Can you work these out from the model? Positions are in its coordinate system, mm. A direction names the side the tool comes from. Round coordinates to 2 decimals unless told otherwise and drop trailing zeros. Write each loop counter-clockwise with the first axis right and the second up, starting at its lowest first coordinate (ties: lowest second). Pieces come first, ordered by that corner, then holes. Notation, with made-up numbers: M 27,76 L 41,76 A11 cw 41,94 Z; hole C 55,-29 d8. An arc over 180 degrees is marked long. Answer in a Markdown table with one row per item. Add a question column.
(1) If we mould it in two halves opening along Z, with no side actions, what happens to faces 1 (the face through (-39, 20.1, 10)), 2 (the face through (-15, 10, -2))? For each: released by +Z, released by -Z, zero draft, split by the parting line, or undercut.
(2) Suppose I cut it at D-D, the plane y = 22.25. Write out the boundary of the cut face in (x, z), then the cut area to 3 significant figures.
(3) Suppose I cut it at C-C, the plane x = -17.5. Write out the boundary of the cut face in (y, z).
(4) If I drill on probe 1 along Y at (x, z) = (-59, 19.25); probe 2 along Z at (x, y) = (-62, 2.5), over which ranges is the centre line in solid material (lowest first)?
(5) Suppose I cut it at B-B, the plane y = 10.05. Write out the boundary of the cut face in (x, z), then the cut area to 3 significant figures.
(6) Suppose I cut it at A-A, the plane z = 10.05. Write out the boundary of the cut face in (x, y).
(7) For faces 3 (the face through (-39.44, 4.48, 13.97)), 4 (the face through (-6, 22, 13.05)), 5 (the face through (-6, 7.05, -2)), 6 (the face through (-39, -4, 10)), 7 (the face through (-39, 24.1, 10)), which set-ups out of +Z, -Z, +X, -X, +Y, -Y let a thin tool reach every point of the face, with its end or its side?
Autodesk Inventor part; units mm, degrees
ref_plane "YZ Plane" through (0, 0, 0) normal (1, 0, 0) x (0, 1, 0)
ref_plane "XZ Plane" through (0, 0, 0) normal (0, 1, 0) x (-1, 0, 0)
ref_plane "XY Plane" through (0, 0, 0) normal (0, 0, 1) x (1, 0, 0)
sketch "Sketch1" plane through (0, 0, 0) normal (1, 0, 0) x (0, 1, 0)
  line L0 (0, 0) -> (20.1, 0)
  line L1 (20.1, 0) -> (20.1, 20.1)
  line L2 (20.1, 20.1) -> (0, 20.1)
  line L3 (0, 20.1) -> (0, 0)
  line L4 (-4, 24.1) -> (24.1, 24.1)
  line L5 (24.1, 24.1) -> (24.1, -4)
  line L6 (24.1, -4) -> (-4, -4)
  line L7 (-4, -4) -> (-4, 24.1)
  line L8 (12.55, 22.2) -> (7.55, 22.2)
  line L9 (7.55, 22.2) -> (7.55, 18)
  line L10 (7.55, 18) -> (12.55, 18)
  line L11 (12.55, 18) -> (12.55, 22.2)
  line L12 (12.55, 22.2) -> (7.55, 18) construction
  line L13 (7.55, 22.2) -> (12.55, 18) construction
  line L14 (12.55, 18) -> (15.35, 18)
  line L15 (15.35, 18) -> (15.35, 17)
  line L16 (15.35, 17) -> (12.55, 14.2)
  line L17 (12.55, 14.2) -> (7.55, 14.2)
  line L18 (7.55, 18) -> (4.75, 18)
  line L19 (4.75, 18) -> (4.75, 17)
  line L20 (4.75, 17) -> (7.55, 14.2)
  line L21 (2.1, 15.35) -> (3.1, 15.35)
  line L22 (3.1, 4.75) -> (5.9, 7.55)
  line L23 (2.1, 4.75) -> (3.1, 4.75)
  line L24 (-2.1, 12.55) -> (-2.1, 7.55)
  line L25 (2.1, 12.55) -> (-2.1, 12.55)
  line L26 (-2.1, 12.55) -> (2.1, 7.55) construction
  line L27 (-2.1, 7.55) -> (2.1, 12.55) construction
  line L28 (2.1, 7.55) -> (2.1, 4.75)
  line L29 (-2.1, 7.55) -> (2.1, 7.55)
  line L30 (2.1, 7.55) -> (2.1, 12.55)
  line L31 (5.9, 12.55) -> (5.9, 7.55)
  line L32 (2.1, 12.55) -> (2.1, 15.35)
  line L33 (3.1, 15.35) -> (5.9, 12.55)
  point P0 (10.05, 20.1)
  point P1 (0, 10.05)
  point P2 (10.05, 20.1)
  point P3 (0, 10.05)
  point P4 (0, 7.55)
  point P5 (0, 12.55)
  point P6 (7.55, 20.1)
  point P7 (12.55, 20.1)
  dimension "d0" = 20.1
  dimension "d1" = 20.1
  dimension "d2" = 4
  dimension "d3" = 5
  dimension "d4" = 4.2
  dimension "d5" = 2.8
  dimension "d6" = 1
  dimension "d7" = 3.8
  dimension "d8" = 2.8
  dimension "d9" = 5
  dimension "d10" = 1
  dimension "d11" = 135
  dimension "d12" = 5
  dimension "d13" = 4.2
  dimension "d14" = 2.8
  dimension "d15" = 1
  dimension "d16" = 3.8
  dimension "d17" = 2.8
  dimension "d18" = 5
  dimension "d19" = 1
  dimension "d20" = 135
  dimension "d21" = 7.55
  dimension "d22" = 2.1
  dimension "d23" = 90
  dimension "d24" = 7.55
  dimension "d25" = 2.1
  dimension "d26" = 90
extrude "Extrusion1" add sketch "Sketch1" against normal blind 80 contours L29 L24 L25 L3 | L3 L25 L30 L29 | L30 L32 L21 L33 L31 L22 L23 L28 | L11 L10 L9 L2 | L2 L9 L8 L11 | L14 L15 L16 L17 L20 L19 L18 L10 | L4 L5 L6 L7
sketch "Sketch2" plane through (0, -4, -4) normal (0, -1, 0) x (1, 0, 0)
  line L0 (0, 28.1) -> (0, 0)
  line L1 (0, 28.1) -> (-80, 28.1)
  line L2 (-80, 0) -> (-80, 28.1)
  line L3 (0, 0) -> (-80, 0)
  line L4 (-80, 0) -> (0, 28.1) construction
  line L5 (-80, 28.1) -> (0, 0) construction
  line L6 (-60.4, 34.15) -> (-60.4, -6.05) construction
  line L7 (-60.4, -6.05) -> (-19.6, -6.05) construction
  line L8 (-19.6, -6.05) -> (-19.6, 34.15) construction
  line L9 (-19.6, 34.15) -> (-60.4, 34.15) construction
  line L10 (-60.4, 34.15) -> (-19.6, -6.05) construction
  line L11 (-60.4, -6.05) -> (-19.6, 34.15) construction
  circle A0 centre (-19.6, 34.15) radius 1.6
  circle A1 centre (-19.6, -8.25) radius 1.6
  circle A2 centre (-57.6, 34.15) radius 1.6
  circle A3 centre (-57.6, -8.25) radius 1.6
  line L12 (-23, 28.1) -> (-57, 28.1)
  line L13 (-23, 0) -> (-57, 0)
  line L14 (0, 28.1) -> (-80, 28.1)
  point P0 (0, 4)
  point P1 (-40, 14.05)
  dimension "d32" = 3.2
  dimension "d35" = 42.4
  dimension "d38" = 38
  dimension "d66" = 40.8
  dimension "d67" = 40.2
extrude "Extrusion2" [suppressed]
sketch "Sketch3" plane through (0, 24.1, 24.1) normal (0, 1, 0) x (1, 0, 0)
  line L0 (0, 28.1) -> (0, 0)
  line L1 (0, 28.1) -> (-80, 28.1)
  line L2 (-80, 0) -> (-80, 28.1)
  line L3 (0, 0) -> (-80, 0)
  line L4 (0, 16.55) -> (0, 11.55) construction
  line L5 (0, 14.05) -> (-80, 14.05) construction
  line L6 (-80, 28.1) -> (-80, 0) construction
  circle A0 centre (-12, 14.05) radius 3
  circle A1 centre (-68, 14.05) radius 3
  line L7 (-68, 17.05) -> (-80, 17.05)
  line L8 (-68, 11.05) -> (-80, 11.05)
  line L9 (-12, 17.05) -> (0, 17.05)
  line L10 (0, 19.35) -> (0, 16.55)
  line L11 (-12, 11.05) -> (0, 11.05)
  line L12 (0, 8.75) -> (0, 11.55)
  point P0 (0, 24.1)
  point P1 (0, 11.05)
  point P2 (-80, 11.05)
  dimension "d49" = 6
  dimension "d50" = 6
  dimension "d51" = 12
  dimension "d52" = 12
  dimension "d53" = 6
  dimension "d54" = 6
extrude "Extrusion3" cut sketch "Sketch3" against normal up to surface (4 mm away) contours L0 L11 A0 L9 | L7 A1 L8 L2 | A0 | A1
ref_plane "Work Plane1" through (0, 24.1, -4) normal (0, -0.7071, -0.7071) x (-1, 0, 0)
mirror "Mirror1" about plane through (0, 24.1, -4) normal (0, -0.7071, -0.7071) of "Extrusion3"
extrude "Extrusão4" [suppressed]
fillet "Arredondamento3" [suppressed]
equation "\"d8\" = d5"
equation "\"d9\" = d3"
equation "\"d10\" = d6"
equation "\"d17\" = d14"
equation "\"d18\" = d12"
equation "\"d19\" = d15"
properties part number "cameraSlider3"
Calculated:
| question | item | result |
|---|---|---|
| 1 | face 1 | undercut |
| 1 | face 2 | zero draft |
| 2 | outline | M -80,-4 L 0,-4 L 0,7.05 L -12,7.05 A3 cw -12,13.05 L 0,13.05 L 0,24.1 L -80,24.1 L -80,13.05 L -68,13.05 A3 cw -68,7.05 L -80,7.05 Z |
| 2 | area | 2,080 mm² |
| 3 | outline | M -4,-4 L 24.1,-4 L 24.1,24.1 L -4,24.1 Z; hole M 0,0 L 20.1,0 L 20.1,20.1 L 12.55,20.1 L 12.55,18 L 15.35,18 L 15.35,17 L 12.55,14.2 L 7.55,14.2 L 4.75,17 L 4.75,18 L 7.55,18 L 7.55,20.1 L 0,20.1 L 0,12.55 L 2.1,12.55 L 2.1,15.35 L 3.1,15.35 L 5.9,12.55 L 5.9,7.55 L 3.1,4.75 L 2.1,4.75 L 2.1,7.55 L 0,7.55 Z |
| 4 | probe 1 | -4 to 0, 7.55 to 12.55, 20.1 to 24.1 |
| 4 | probe 2 | -4 to 0, 4.75 to 15.35, 20.1 to 24.1 |
| 5 | outline | M -80,14.2 L 0,14.2 L 0,24.1 L -80,24.1 Z; M -65,-4 L -15,-4 L -15,0 L -65,0 Z |
| 5 | area | 992 mm² |
| 6 | outline | M -80,-4 L 0,-4 L 0,5.9 L -80,5.9 Z; M -65,20.1 L -15,20.1 L -15,24.1 L -65,24.1 Z |
| 7 | face 3 | +X, -X |
| 7 | face 4 | +X, +Y |
| 7 | face 5 | -Z, +X |
| 7 | face 6 | +Z, -Z, +X, -X, -Y |
| 7 | face 7 | +Z, -Z, +X, -X, +Y |
